Geometry: final body of the model. Coordinates: model frame, mm. A direction names the side the tool comes from. Give positions to 0.01 mm unless a question says otherwise; leave off trailing zeros. Write each loop counter-clockwise with the first axis right and the second up, starting at its lowest first coordinate (ties: lowest second). Pieces come first, ordered by that corner, then holes. Notation, with made-up numbers: M 88,-30.75 L 142,-30.75 A11 ccw 142,-23.75 Z; hole C -35,-26 d11. An arc over 180 degrees is marked long. Answer as a JSON object with one key per item and string values.
from build123d import *

# Parameters (mm, degrees)
SKETCH1_W                    = 25
SKETCH1_H                    = 15
BASE_FLANGE1_DEPTH           = 3.175
EDGE_FLANGE1_STRIP_W         = 14.7
EDGE_FLANGE1_STRIP_H         = 3.175
EDGE_FLANGE1_STRIP_CUT_DEPTH = 15
EDGE_FLANGE1_DEPTH           = 15
M8_CLEARANCE_HOLE2_D         = 9
FILLET1_R                    = 3.175
M4_CLEARANCE_HOLE2_D         = 4.5


# Sheet-metal steps are written as plain solids
with BuildPart() as part:
    # Sketch1 → Base-Flange1 (new body)
    with BuildSketch(Plane.XY):
        Rectangle(SKETCH1_W, SKETCH1_H)
    extrude(amount=BASE_FLANGE1_DEPTH)

    # Edge-Flange1 strip (across the edge) → Edge-Flange1 strip cut (cut)
    with BuildSketch(Plane(origin=(-12.5, 7.5, 3.175), x_dir=(1, 0, 0), z_dir=(0, -1, 0))):
        with Locations((-6.35, -1.5875)):
            Rectangle(EDGE_FLANGE1_STRIP_W, EDGE_FLANGE1_STRIP_H)
    extrude(amount=EDGE_FLANGE1_STRIP_CUT_DEPTH, mode=Mode.SUBTRACT)

    # Edge-Flange1 section (across the edge) → Edge-Flange1 (add)
    with BuildSketch(Plane(origin=(-12.5, 7.5, 3.175), x_dir=(1, 0, 0), z_dir=(0, -1, 0))):
        with BuildLine():
            Line((-3.175, 1), (-3.175, 12.825))
            Line((-3.175, 12.825), (0, 12.825))
            Line((0, 12.825), (0, 1))
            ThreePointArc((0, 1), (0.292893219, 0.292893219), (1, 0))
            Line((1, 0), (1, -3.175))
            ThreePointArc((1, -3.175), (-1.952170811, -1.952170811), (-3.175, 1))
        make_face()
    extrude(amount=EDGE_FLANGE1_DEPTH)

    # M8 Clearance Hole2 (through all)
    with Locations(Plane.XY.offset(3.175)):
        with Locations((4.9369, 0)):
            Hole(M8_CLEARANCE_HOLE2_D / 2)

    # Fillet1
    fillet1_edges = [part.edges().sort_by_distance(p)[0] for p in [
        (-14.0875, 7.5, 16),
        (-14.0875, -7.5, 16),
        (12.5, -7.5, 1.5875),
        (12.5, 7.5, 1.5875),
    ]]
    fillet(fillet1_edges, radius=FILLET1_R)

    # M4 Clearance Hole2 (through all)
    with Locations(Plane(origin=(-12.5, 0, 0), x_dir=(0, 0, -1), z_dir=(1, 0, 0))):
        with Locations((-9, 0)):
            Hole(M4_CLEARANCE_HOLE2_D / 2)


solid = part.part
1) Set-up query: faces 4 (the cylindrical face through (-14.07, 6.55, 15.09)), 5 (the flat face through (-12.5, 0.1, 11.5)). Return all of +Z, -Z, +X, -X, +Y, -Y with unobstructed straight access to the full face (end or side cutting, diameter ignored); none if empty.
Geometry check:
{"face 4": "+Z, +X, -X, +Y", "face 5": "+Z, +X, +Y, -Y"}
2) Cut plane C-C on x = 4. Return loops of the section in (y, z) (3 decimals).
Geometry check:
{"outline": "M -7.5,0 L -4.401,0 L -4.401,3.175 L -7.5,3.175 Z; M 4.401,0 L 7.5,0 L 7.5,3.175 L 4.401,3.175 Z"}
3) Contact query for a flat-ended pin moving along its axis: P1, Ø5, axis at y = -4, z = 13, coming from the +X side. Output: stop coordinate, or through.
Geometry check:
{"P1": "stops at x = -12.5"}
4) Cut plane A-A on z = 9. Return loops of the section in (x, y) (3 decimals), and give its area (3 significant figures).
Geometry check:
{"outline": "M -15.675,-7.5 L -12.5,-7.5 L -12.5,-2.25 L -15.675,-2.25 Z; M -15.675,2.25 L -12.5,2.25 L -12.5,7.5 L -15.675,7.5 Z", "area": "33.3 mm2"}
5) Line query: line 1 (Y direction, x = -14.65, z = 9); line 2 (Z direction, x = 0.25, y = 5) (3 decimals); line 3 (X direction, y = 0.5, z = 6.25) (3 decimals). Output: solid intervals per line, ascending. Write a range as from..to.
Geometry check:
{"line 1": "y = -7.5..-2.25, 2.25..7.5", "line 2": "z = 0..3.175", "line 3": "x = -15.675..-12.5"}
6) Pull-direction query (Z, two-part tool) for faces 1 (the flat face through (-14, 0, 16)), 2 (the cylindrical face through (11.55, -6.59, 1.61)), 3 (the cylindrical face through (-14.11, 0.099, 6.752)); classes: pulls with the +Z half, pulls with the -Z half, needs draft (parallel to the pull), parting line crosses it, or undercut.
Geometry check:
{"face 1": "pulls with the +Z half", "face 2": "needs draft", "face 3": "undercut"}
7) Cut plane D-D on y = 3. Return loops of the section in (x, z) (3 decimals).
Geometry check:
{"outline": "M -15.675,4.175 A4.175 ccw -11.5,0 L 1.583,0 L 1.583,3.175 L -11.5,3.175 A1 cw -12.5,4.175 L -12.5,16 L -15.675,16 Z; M 8.291,0 L 12.5,0 L 12.5,3.175 L 8.291,3.175 Z"}
8) Cut plane B-B on y = 0. Return loops of the section in (x, z) (3 decimals), and give its area (3 significant figures).
Geometry check:
{"outline": "M -15.675,4.175 A4.175 ccw -11.5,0 L 0.437,0 L 0.437,3.175 L -11.5,3.175 A1 cw -12.5,4.175 L -12.5,6.75 L -15.675,6.75 Z; M -15.675,11.25 L -12.5,11.25 L -12.5,16 L -15.675,16 Z; M 9.437,0 L 12.5,0 L 12.5,3.175 L 9.437,3.175 Z", "area": "83.8 mm2"}
